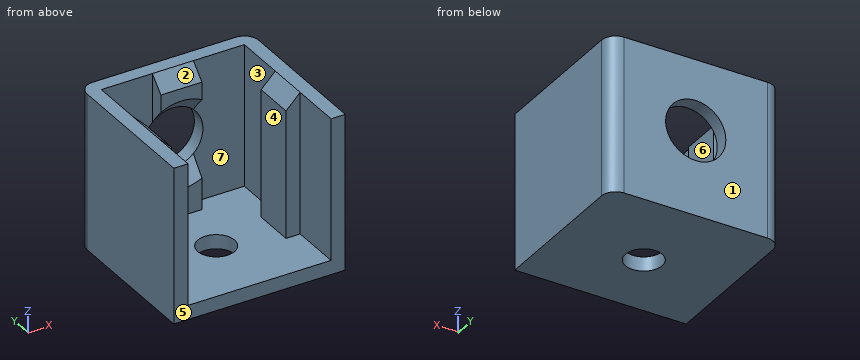
from build123d import *

# Parameters (mm, degrees)
F1_W      = 5.8
F1_H      = 2
F2_DEPTH  = 20
F4_COUNT  = 4
F5_R      = 4.25
F6_DEPTH  = 24.201
F8_DEPTH  = 20.001
F9_W      = 24.2
F9_H      = 22.2
F9_R      = 2.6
F10_DEPTH = 2
F11_R     = 2
F12_SIZE  = 2


with BuildPart() as f2:
    # F1 (on Top) → F2 (new body)
    with BuildSketch(Plane.XY):
        Polygon((-12.1, 12.1), (-12.1, 10.1), (-2.9, 10.1), (2.9, 10.1), (12.1, 10.1), (12.1, 12.1), align=None)
        with Locations((0, 9.1)):
            Rectangle(F1_W, F1_H)
    extrude(amount=F2_DEPTH)

    # F4: F2 ×4 about axis
    f4_axis = Axis((0, 0, 13.2065918297), (0, 0, 1))


with BuildPart() as f2_1:
    add(f2.part)
    for i in range(1, F4_COUNT):
        add(f2.part.rotate(f4_axis, i * 360 / F4_COUNT))

    # F5 (on face) → F6 (cut, through all)
    with BuildSketch(Plane(origin=(0, 12.1, 0), x_dir=(-1, 0, 0), z_dir=(0, 1, 0))):
        with Locations((0, 10)):
            Circle(F5_R)
    extrude(amount=-F6_DEPTH, mode=Mode.SUBTRACT)

    # F7 (on face) → F8 (cut, through all)
    with BuildSketch(Plane.XY.offset(20)):
        Polygon((-2.9, -8.1), (-10.1, -10.1), (-12.1, -10.1), (-12.1, -12.1), (12.1, -12.1), (12.1, -10.1), (10.1, -10.1), (2.9, -8.1), align=None)
    extrude(amount=-F8_DEPTH, mode=Mode.SUBTRACT)

    # F9 (on face) → F10 (join)
    with BuildSketch(Plane(origin=(0, 0, 0), x_dir=(1, 0, 0), z_dir=(0, 0, -1))):
        with Locations((0, -1)):
            Rectangle(F9_W, F9_H)
        Circle(F9_R, mode=Mode.SUBTRACT)
    extrude(amount=F10_DEPTH)

    # F11
    f11_edges = [f2_1.edges().sort_by_distance(p)[0] for p in [
        (-12.1, 12.1, 9),
        (12.1, 12.1, 9),
    ]]
    fillet(f11_edges, radius=F11_R)

    # F12
    f12_edges = [f2_1.edges().sort_by_distance(p)[0] for p in [
        (0, 8.1, 5.75),
        (0, 8.1, 14.25),
        (-8.1, 0, 20),
        (0, 8.1, 20),
        (8.1, 0, 20),
    ]]
    chamfer(f12_edges, length=F12_SIZE)


solid = f2_1.part
Read the model definition and answer for the solid it produces. Units are mm, in the model's axes. Face numbers are marked on the shaded views. A direction names the side the tool comes from. Give positions to 0.01 mm unless a question says otherwise; leave off trailing zeros. Loops run counter-clockwise (first coordinate to the right, second up) from the corner with the lowest first, then second, coordinate; pieces in that order, holes last. Notation, with made-up numbers: (8, -35.75) - (63, -35.75) arc R23 cw to (63, -17.75) - close; hole circle Ø8 at (31.25, 28). An arc over 180 degrees is marked (long way). Answer as CSV lines item,"result". Start each with the question number.
1) Which of the six approach directions +Z, -Z, +X, -X, +Y, -Y give full straight-line access (tool end or side, diameter ignored) to the marked faces 5, 6 and 7?
2) Find section B-B (z = 10). Write down the section's boundary in (x, y), then the cut area to 3 significant figures.
3) Determine the mould class of the marked faces 1, 2, 3 and 4 for opening direction Y: released by +Y, released by -Y, zero draft, split by the parting line, or undercut.
4) Find section A-A (y = 0). Write down the section's boundary in (x, z).
5) Straight lines are drawn through the part: L1, parallel to X at y = -3, z = 8.25; L2, parallel to Z at x = 0, y = 11.35; L3, parallel to Y at x = -9.5, z = 11.25. For each, find the intervals that lie inside material, in ascending order. Write a range as from..to.
6) Find section C-C (x = 0). Write down the section's boundary in (y, z).
7) Find section D-D (y = 7.5). Write down the section's boundary in (x, z).
8) Each of these flat-tipped pins is pushed along its axis until it touches: pin 1 Ø2.5 at (x, z) = (1, 16.5) entering from -Y; pin 2 Ø2 at (x, z) = (3.5, 10.5) entering from -Y; pin 3 Ø0.6 at (x, z) = (-9, 6.5) entering from -Y. Where does it stop, or does it pass through?
Findings below:
1,face 5,"+Z, -Z, +X, -X, -Y"
1,face 6,"+Z, -Y"
1,face 7,"+Z"
2,outline,"(-12.1, -10.1) - (-10.1, -10.1) - (-10.1, -2.9) - (-8.1, -2.9) - (-8.1, 2.9) - (-10.1, 2.9) - (-10.1, 10.1) - (-4.25, 10.1) - (-4.25, 12.1) - (-10.1, 12.1) arc R2 ccw to (-12.1, 10.1) - close; (4.25, 10.1) - (10.1, 10.1) - (10.1, 2.9) - (8.1, 2.9) - (8.1, -2.9) - (10.1, -2.9) - (10.1, -10.1) - (12.1, -10.1) - (12.1, 10.1) arc R2 ccw to (10.1, 12.1) - (4.25, 12.1) - close"
2,area,"134 mm^2"
3,face 1,"released by +Y"
3,face 2,"released by -Y"
3,face 3,"undercut"
3,face 4,"zero draft"
4,outline,"(-12.1, -2) - (-2.6, -2) - (-2.6, 0) - (-8.1, 0) - (-8.1, 18) - (-10.1, 20) - (-12.1, 20) - close; (2.6, -2) - (12.1, -2) - (12.1, 20) - (10.1, 20) - (8.1, 18) - (8.1, 0) - (2.6, 0) - close"
5,L1,"-12.1..-10.1, 10.1..12.1"
5,L2,"-2..5.75, 14.25..20"
5,L3,"-2.9..2.9, 10.1..12.1"
6,outline,"(-10.1, -2) - (-2.6, -2) - (-2.6, 0) - (-10.1, 0) - close; (2.6, -2) - (12.1, -2) - (12.1, 5.75) - (10.1, 5.75) - (8.1, 3.75) - (8.1, 0) - (2.6, 0) - close; (8.1, 16.25) - (10.1, 14.25) - (12.1, 14.25) - (12.1, 20) - (10.1, 20) - (8.1, 18) - close"
7,outline,"(-12.1, -2) - (12.1, -2) - (12.1, 20) - (10.1, 20) - (10.1, 0) - (-10.1, 0) - (-10.1, 20) - (-12.1, 20) - close"
8,pin 1,"y = 8.1"
8,pin 2,"y = 10.1"
8,pin 3,"y = -2.9"
